Check sheet for the modelled part. Datum: model origin and axes. Units: mm. Round coordinates to 2 decimals unless told otherwise and drop trailing zeros. Write each loop counter-clockwise with the first axis right and the second up, starting at its lowest first coordinate (ties: lowest second). Pieces come first, ordered by that corner, then holes. Notation, with made-up numbers: (57, 15.25) -> (112, 15.25) arc R29 cw to (112, 38.25) -> close; hole circle Ø6 at (78.25, 0.5). An arc over 180 degrees is marked (long way). Answer as a JSON object with one key per item and string values. Group by question number.
Autodesk Inventor part; units mm, degrees
ref_plane "YZ Plane" through (0, 0, 0) normal (1, 0, 0) x (0, 1, 0)
ref_plane "XZ Plane" through (0, 0, 0) normal (0, 1, 0) x (-1, 0, 0)
ref_plane "XY Plane" through (0, 0, 0) normal (0, 0, 1) x (1, 0, 0)
sketch "Sketch1" plane through (0, 0, 0) normal (0, 1, 0) x (-1, 0, 0)
  circle A0 centre (0, 0) radius 79.375
  circle A1 centre (0, 0) radius 177.8
  dimension "d0" = 158.75
  dimension "d1" = 355.6
extrude "Extrusion1" add sketch "Sketch1" along normal blind 0.6
sketch "Sketch2" plane through (0, 0.6, 0) normal (0, 1, 0) x (1, 0, 0)
  point P0 (0, 0)
  point P1 (0, 90.4875)
  point P2 (-70.746, 56.418)
  point P3 (-88.2188, -20.1354)
  point P4 (-39.2611, -81.5264)
  point P5 (39.2611, -81.5264)
  point P6 (88.2188, -20.1354)
  point P7 (70.746, 56.418)
  dimension "d4" = 90.4875
  dimension "d7" = 360
hole "Hole1" at (0, 0.6, -90.4875) at (-70.746, 0.6, -56.418) at (-88.2188, 0.6, 20.1354) at (-39.2611, 0.6, 81.5264) at (39.2611, 0.6, 81.5264) at (88.2188, 0.6, 20.1354) at (70.746, 0.6, -56.418) direction (0, -1, 0) diameter 6.7564 end through all
sketch "Sketch3" plane through (0, 0.6, 0) normal (0, 1, 0) x (1, 0, 0)
  point P0 (0, 0)
  point P1 (-143.51, 0)
  dimension "d16" = 143.51
hole "Hole2" at (-143.51, 0.6, 0) direction (0, -1, 0) diameter 31.75 end through all
properties part number "3DPRINT,WIRE-GUARD"
(1) Scan lines: line 1 along Z through (x, y) = (0, 0.4) (3 decimals); line 2 along Z through (x, y) = (69, 0.1); line 3 along X through (y, z) = (0.4, 23). Record each from-to range of solid material in increasing order.
(2) Section check A-A on z = 0. Record the cut outline in (x, y) (3 decimals), then the cut area to 3 significant figures.
(3) Section check B-B on x = -57.5. Record the cut outline in (y, z), then the cut area to 3 significant figures.
(4) Release check for a two-part mould opening along X. For faces 1 (the cylindrical face through (-169.59, 0.3, -53.41)), 2 (the flat face through (-37, 0.6, -77)), 3 (the cylindrical face through (-75.71, 0.3, -23.84)) record: pulls with the +X half, pulls with the -X half, needs draft (parallel to the pull), parting line crosses it, or undercut.
(5) Section check C-C on z = -68. Record the cut outline in (x, y), then the cut area to 3 significant figures.
(6) Go/stop test with a flat-tipped pin: pin 1 Ø4 at (x, z) = (-88.22, 20.14) entering from -Y. Record where the tip stops, or that it passes through.
(7) Section check D-D on y = 0.4. State how many separate pieces and enclosed holes the cut face has, then the cut area to 3 significant figures.
Data:
{
 "1": {"line 1": "z = -177.8 to -93.866, -87.109 to -79.375, 79.375 to 177.8", "line 2": "z = -163.87 to -59.31, -53.53 to -39.24, 39.24 to 163.87", "line 3": "x = -176.31 to -90.01, -86.43 to -75.97, 75.97 to 86.43, 90.01 to 176.31"},
 "2": {"outline": "(-177.8, 0) -> (-159.385, 0) -> (-159.385, 0.6) -> (-177.8, 0.6) -> close; (-127.635, 0) -> (-79.375, 0) -> (-79.375, 0.6) -> (-127.635, 0.6) -> close; (79.375, 0) -> (177.8, 0) -> (177.8, 0.6) -> (79.375, 0.6) -> close", "area": "99.1 mm²"},
 "3": {"outline": "(0, -168.25) -> (0.6, -168.25) -> (0.6, -54.72) -> (0, -54.72) -> close; (0, 54.72) -> (0.6, 54.72) -> (0.6, 168.25) -> (0, 168.25) -> close", "area": "136 mm²"},
 "4": {"face 1": "parting line crosses it", "face 2": "needs draft", "face 3": "undercut"},
 "5": {"outline": "(-164.28, 0) -> (-40.94, 0) -> (-40.94, 0.6) -> (-164.28, 0.6) -> close; (40.94, 0) -> (164.28, 0) -> (164.28, 0.6) -> (40.94, 0.6) -> close", "area": "148 mm²"},
 "6": {"pin 1": "passes through"},
 "7": {"separate pieces": "1", "enclosed holes": "9", "area": "78,500 mm²"}
}
